from build123d import *

# Parameters (mm, degrees)
SKETCH1_W           = 5.5
SKETCH1_H           = 8
BOSS_EXTRUDE1_DEPTH = 2
SLOT_TAB_DEPTH      = 2
DEBURS_SIZE         = 0.2


with BuildPart() as part:
    # Sketch1 → Boss-Extrude1 (new body)
    with BuildSketch(Plane.XY):
        Rectangle(SKETCH1_W, SKETCH1_H)
    extrude(amount=-BOSS_EXTRUDE1_DEPTH)

    # Sketch2 → Slot Tab (add)
    with BuildSketch(Plane.XY):
        with BuildLine():
            ThreePointArc((-2.142428529, 4), (0, 2.3), (2.142428529, 4))
            Line((2.142428529, 4), (-2.142428529, 4))
        make_face()
    slot_tab = extrude(amount=SLOT_TAB_DEPTH)

    # Slot Tabs: Slot Tab across plane
    add(slot_tab.mirror(Plane.ZX))

    # Deburs
    deburs_edges = [part.edges().sort_by_distance(p)[0] for p in [
        (-2.75, 0, -2),
        (0, 2.3, 2),
        (0, -4, -2),
        (0, -2.3, 2),
        (2.75, 0, -2),
        (2.75, -4, -1),
        (-2.75, -4, -1),
        (-2.75, 4, -1),
        (2.75, 4, -1),
        (0, 4, -2),
    ]]
    chamfer(deburs_edges, length=DEBURS_SIZE)


solid = part.part
Input: part model. Units: mm. Frame: model coordinates. Coordinates: 2 decimals unless noted, no trailing zeros. Order: outer loops, then holes, each group sorted by start corner. A loop starts at its lowest first (then second) coordinate and runs counter-clockwise, first axis right, second up. Notation, with made-up numbers: M 4.25,-17 L 11.25,-17 A9 ccw 11.25,0 Z; hole C 21,66 d1. An arc over 180 degrees is marked long. Answer in a Markdown table with one row per item.
(1) Material intervals for line 1 (Y direction, x = 0.05, z = 0.6); line 2 (Z direction, x = 0.8, y = -2); line 3 (Y direction, x = -0.9, z = 1.7), sorted ascending. Write a range as [from, to].
Numbers:
| item | result |
|---|---|
| line 1 | y = [-4, -2.3], [2.3, 4] |
| line 2 | z = [-2, 0] |
| line 3 | y = [-4, -2.49], [2.49, 4] |
(2) Section query A-A, the plane z = 0.2. Output: boundary loops of the cut face in (x, y), plus the area to 3 significant figures.
Numbers:
| item | result |
|---|---|
| outline | M -2.14,-4 L 2.14,-4 A2.2 ccw Z; M -2.14,4 A2.2 ccw 2.14,4 Z |
| area | 10.8 mm^2 |
(3) Section query B-B, the plane y = 2. Output: boundary loops of the cut face in (x, z), plus the area to 3 significant figures.
Numbers:
| item | result |
|---|---|
| outline | M -2.75,-1.8 L -2.55,-2 L 2.55,-2 L 2.75,-1.8 L 2.75,0 L -2.75,0 Z |
| area | 11.0 mm^2 |
(4) Draft query along Y for faces 1 (the flat face through (2.75, 0, -1)), 2 (the cylindrical face through (0, 2.3, 0.9)), 3 (the cylindrical face through (0, -2.3, 0.9)), 4 (the flat face through (0, -4, 0)). Return one class per face: pulls with the +Y half, pulls with the -Y half, needs draft (parallel to the pull), parting line crosses it, or undercut.
Numbers:
| item | result |
|---|---|
| face 1 | needs draft |
| face 2 | undercut |
| face 3 | undercut |
| face 4 | pulls with the -Y half |
